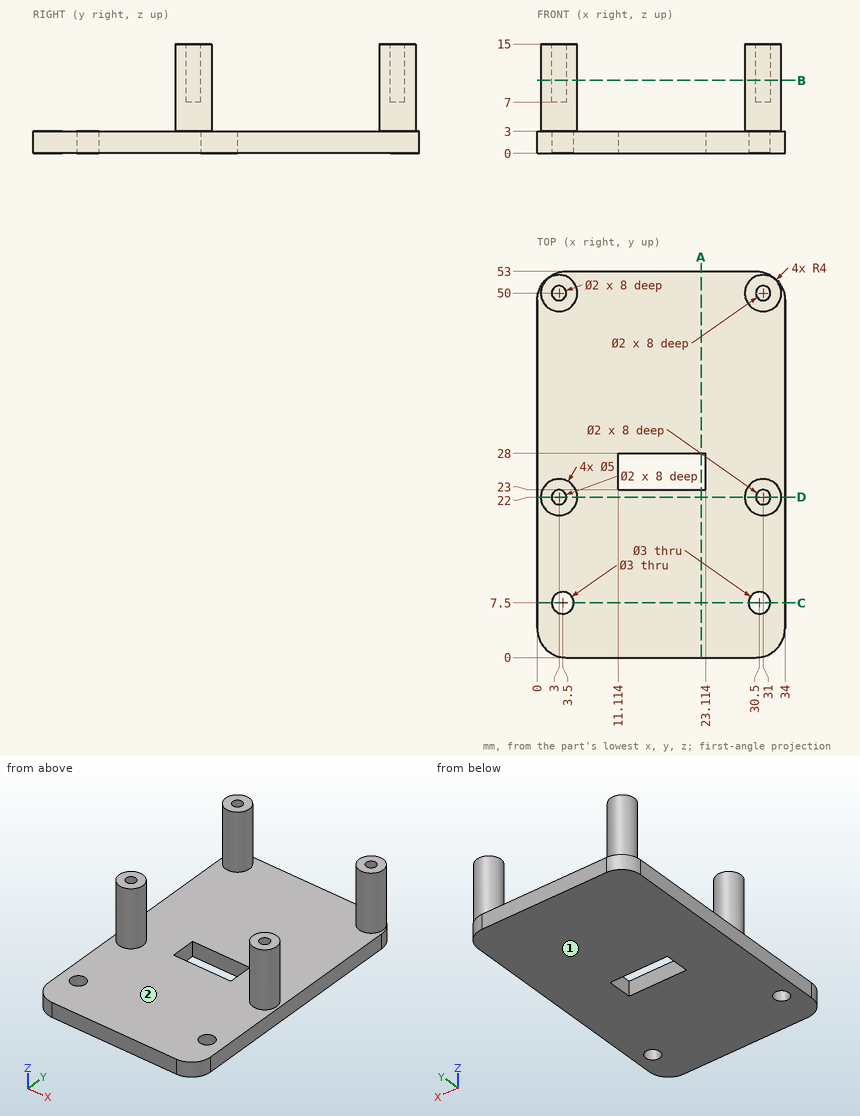
Check sheet for the drawn part. Datum: minimum x, y, z corner. Units: mm. Round coordinates to 2 decimals unless told otherwise and drop trailing zeros. Write each loop counter-clockwise with the first axis right and the second up, starting at its lowest first coordinate (ties: lowest second). Pieces come first, ordered by that corner, then holes. Notation, with made-up numbers: (-18, 55.25) -> (21, 55.25) arc R16 ccw to (21, 63.25) -> close; hole circle Ø6 at (-29, 27.5). An arc over 180 degrees is marked (long way). Write each question's results on one line, items separated by ' | '.
Q1. Draft check along Y on the marked faces 1 and 2. Enter one of: released by +Y, released by -Y, zero draft, split by the parting line, or undercut.
Derived:
face 1: zero draft | face 2: undercut
Q2. Thickness scan on probe 1 along Y at (x, z) = (31, 12); probe 2 along Y at (x, z) = (20.5, 2.25); probe 3 along Z at (x, y) = (25, 18.5). Record the ranges inside material, lowest first.
Derived:
probe 1: y = 19.5 to 21, 23 to 24.5, 47.5 to 49, 51 to 52.5 | probe 2: y = 0 to 23, 28 to 53 | probe 3: z = 0 to 3
Q3. Sectioned sample at A-A, the plane x = 22.5. Record the boundary of the cut face in (y, z).
Derived:
outline: (0, 0) -> (23, 0) -> (23, 3) -> (0, 3) -> close; (28, 0) -> (53, 0) -> (53, 3) -> (28, 3) -> close
Q4. Sectioned sample at C-C, the plane y = 7.5. Record the boundary of the cut face in (x, z), and give its area (3 significant figures).
Derived:
outline: (0, 0) -> (2, 0) -> (2, 3) -> (0, 3) -> close; (5, 0) -> (29, 0) -> (29, 3) -> (5, 3) -> close; (32, 0) -> (34, 0) -> (34, 3) -> (32, 3) -> close | area: 84.0 mm²
Q5. Go/stop test with flat-tipped pins: pin 1 Ø2.5 at (x, y) = (30.5, 7.5) entering from +Z; pin 2 Ø5 at (x, y) = (3.5, 7.5) entering from +Z; pin 3 Ø0.6 at (x, y) = (31, 22) entering from +Z. Record where each tip stops, or that it passes through.
Derived:
pin 1: passes through | pin 2: stops at z = 3 | pin 3: stops at z = 7
Q6. Sectioned sample at B-B, the plane z = 10. Record the boundary of the cut face in (x, y).
Derived:
outline: circle Ø5 at (3, 22); circle Ø5 at (3, 50); circle Ø5 at (31, 22); circle Ø5 at (31, 50); hole circle Ø2 at (3, 22); hole circle Ø2 at (3, 50); hole circle Ø2 at (31, 22); hole circle Ø2 at (31, 50)
Q7. Sectioned sample at D-D, the plane y = 22. Record the boundary of the cut face in (x, z), and give its area (3 significant figures).
Derived:
outline: (0, 0) -> (34, 0) -> (34, 3) -> (33.5, 3) -> (33.5, 15) -> (32, 15) -> (32, 7) -> (30, 7) -> (30, 15) -> (28.5, 15) -> (28.5, 3) -> (5.5, 3) -> (5.5, 15) -> (4, 15) -> (4, 7) -> (2, 7) -> (2, 15) -> (0.5, 15) -> (0.5, 3) -> (0, 3) -> close | area: 190 mm²
